Geometry: see drawing. Coordinates: mm, zero at the bounding-box minimum. A direction names the side the tool comes from. Round coordinates to 2 decimals unless told otherwise and drop trailing zeros. Write each loop counter-clockwise with the first axis right and the second up, starting at its lowest first coordinate (ties: lowest second). Pieces come first, ordered by that corner, then holes. Notation, with made-up numbers: (43.25, -5) -> (83.25, -5) arc R36 cw to (83.25, 34) -> close; hole circle Ø8 at (7, 29). An arc over 180 degrees is marked (long way). Write item = value, one per line.
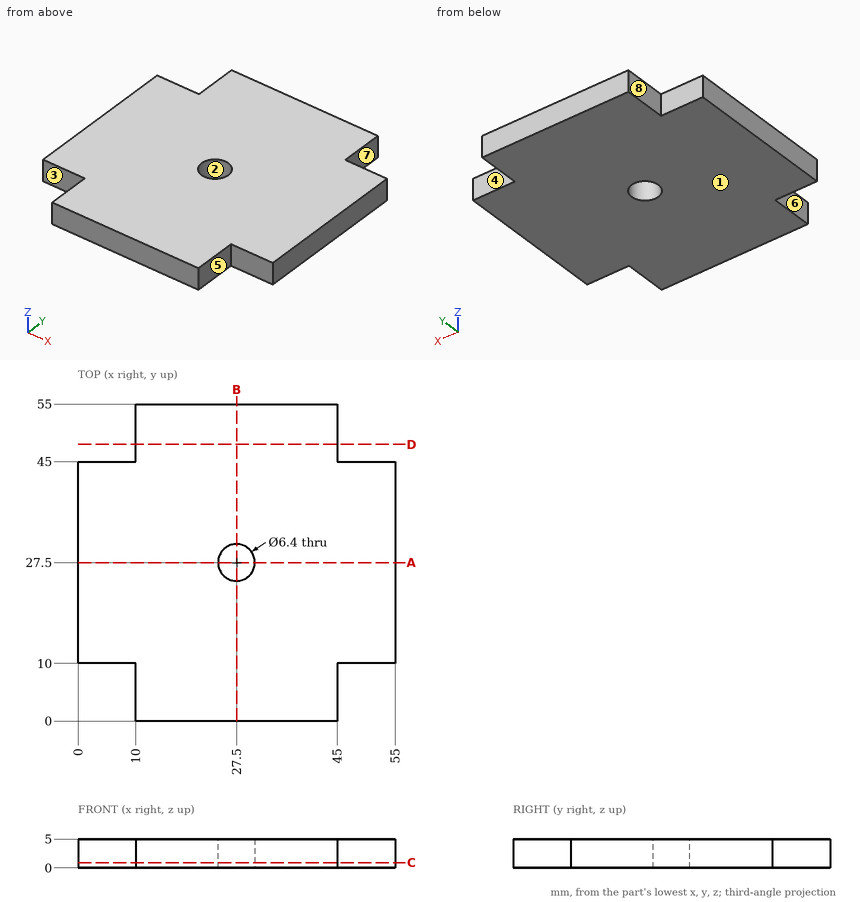
1) Cut plane C-C (z = 0.9). Return the cut outline in (x, y).
Solutions:
outline = (0, 10) -> (10, 10) -> (10, 0) -> (45, 0) -> (45, 10) -> (55, 10) -> (55, 45) -> (45, 45) -> (45, 55) -> (10, 55) -> (10, 45) -> (0, 45) -> close; hole circle Ø6.4 at (27.5, 27.5)
2) Access query for the marked faces 5, 6, 7 and 8. Directions: +Z, -Z, +X, -X, +Y, -Y. A direction counts if a zero-diameter tool reaches every point of the face in a straight line with its end or side. Return the directions, or none.
Solutions:
face_5 = +Z, -Z, +X, -Y
face_6 = +Z, -Z, -X, -Y
face_7 = +Z, -Z, +X, +Y
face_8 = +Z, -Z, -X, +Y
3) First-contact query: P1, Ø1.5, axis at y = 4, z = 3, coming from the +X side; P2, Ø1.5, axis at y = 49.5, z = 2, coming from the -X side. Flat tips, straight axial feed; report the tip coordinate or a pass-through.
Solutions:
P1 = 45
P2 = 10
4) Cut plane A-A (y = 27.5). Return the cut outline in (x, z), and give its area (3 significant figures).
Solutions:
outline = (0, 0) -> (24.3, 0) -> (24.3, 5) -> (0, 5) -> close; (30.7, 0) -> (55, 0) -> (55, 5) -> (30.7, 5) -> close
area = 243 mm^2
5) Line query: L1, parallel to Y at x = 27.5, z = 1.9; L2, parallel to Y at x = 7.5, z = 3.55. Output: solid intervals per line, ascending. Write a range as from..to.
Solutions:
L1 = 0..24.3, 30.7..55
L2 = 10..45
6) Draft query along Y for the marked faces 1, 2, 3 and 4. Return one class per face: +Y half, -Y half, draft (parallel to the pull), parting line (faces both ways), or undercut.
Solutions:
face_1 = draft
face_2 = undercut
face_3 = -Y half
face_4 = +Y half
7) Cut plane D-D (y = 48). Return the cut outline in (x, z), and give its area (3 significant figures).
Solutions:
outline = (10, 0) -> (45, 0) -> (45, 5) -> (10, 5) -> close
area = 175 mm^2
